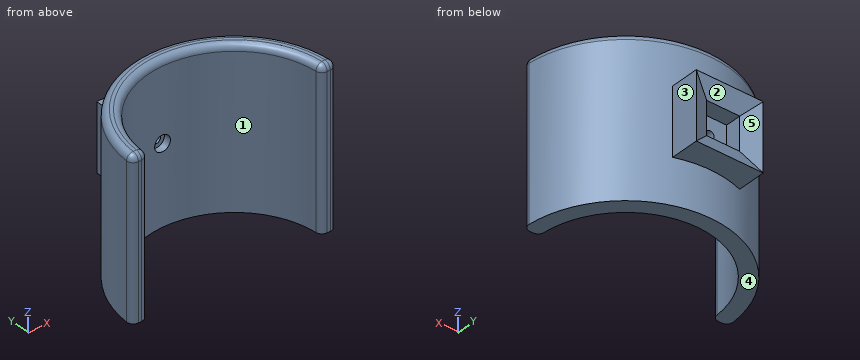
from build123d import *
from OCP.BRepFilletAPI import BRepFilletAPI_MakeChamfer

# Parameters (mm, degrees)
BOSS_EXTRUDE1_DEPTH = 50
BOSS_EXTRUDE2_DEPTH = 21.25
FILLET1_R           = 4
FILLET2_R           = 4
SKETCH3_W           = 21
SKETCH3_H           = 21
CUT_EXTRUDE1_DEPTH  = 15
CHAMFER1_SIZE       = 5
CHAMFER1_SIZE2      = 10.722534603
SKETCH4_R           = 2.5
CUT_EXTRUDE2_DEPTH  = 105.206319677
CUT_EXTRUDE3_START  = -5
SKETCH5_R           = 5
CUT_EXTRUDE3_DEPTH  = 100.206319725


with BuildPart() as part:
    # Sketch1 → Boss-Extrude1 (new, symmetric)
    with BuildSketch(Plane.XY):
        with BuildLine():
            Line((-65, 0), (-55, 0))
            ThreePointArc((-55, 0), (0, 55), (55, 0))
            Line((55, 0), (65, 0))
            ThreePointArc((65, 0), (0, 65), (-65, 0))
        make_face()
    extrude(amount=BOSS_EXTRUDE1_DEPTH, both=True)

    # Sketch2 → Boss-Extrude2 (add, symmetric)
    with BuildSketch(Plane.XY):
        with BuildLine():
            Line((-21.25, 61.428311877), (-21.25, 79.428311877))
            Line((-21.25, 79.428311877), (21.25, 79.428311877))
            Line((21.25, 79.428311877), (21.25, 61.428311877))
            ThreePointArc((21.25, 61.428311877), (0, 65), (-21.25, 61.428311877))
        make_face()
    extrude(amount=BOSS_EXTRUDE2_DEPTH, both=True)

    # Fillet1
    fillet1_edges = [part.edges().sort_by_distance(p)[0] for p in [
        (-55, 0, 0),
        (-65, 0, 0),
        (65, 0, 0),
        (55, 0, 0),
    ]]
    fillet(fillet1_edges, radius=FILLET1_R)

    # Fillet2
    fillet2_edges = [part.edges().sort_by_distance(p)[0] for p in [
        (0, 65, 50),
        (59.866480893, 0, 50),
        (0, 55, 50),
        (-59.866480893, 0, 50),
        (-63.788401254, 1.265880428, 50),
        (-56.133384976, 1.077266197, 50),
        (56.133384976, 1.077266197, 50),
        (63.788401254, 1.265880428, 50),
    ]]
    fillet(fillet2_edges, radius=FILLET2_R)

    # Sketch3 → Cut-Extrude1 (cut)
    with BuildSketch(Plane(origin=(0, 79.428311877, 0), x_dir=(1, 0, 0), z_dir=(0, 1, 0))):
        Rectangle(SKETCH3_W, SKETCH3_H)
    extrude(amount=-CUT_EXTRUDE1_DEPTH, mode=Mode.SUBTRACT)

    # Chamfer1: one chamfer whose edges measure the first distance from different faces: ONE call of the kernel's chamfer builder (chamfer() names one face for all edges)
    chamfer1_edges_1 = [part.edges().sort_by_distance(p)[0] for p in [
        (10.5, 79.428311877, 0),
    ]]
    chamfer1_side_1 = [part.faces().sort_by_distance(p)[0] for p in [
        (10.5, 71.928311877, 0),
    ]]
    chamfer1_edges_2 = [part.edges().sort_by_distance(p)[0] for p in [
        (0, 79.428311877, -10.5),
    ]]
    chamfer1_side_2 = [part.faces().sort_by_distance(p)[0] for p in [
        (0, 71.928311877, -10.5),
    ]]
    chamfer1_edges_3 = [part.edges().sort_by_distance(p)[0] for p in [
        (-10.5, 79.428311877, 0),
    ]]
    chamfer1_side_3 = [part.faces().sort_by_distance(p)[0] for p in [
        (-10.5, 71.928311877, 0),
    ]]
    chamfer1_edges_4 = [part.edges().sort_by_distance(p)[0] for p in [
        (0, 79.428311877, 10.5),
    ]]
    chamfer1_side_4 = [part.faces().sort_by_distance(p)[0] for p in [
        (0, 71.928311877, 10.5),
    ]]
    chamfer1 = BRepFilletAPI_MakeChamfer(part.part.solid().wrapped)
    for e in chamfer1_edges_1:
        chamfer1.Add(CHAMFER1_SIZE, CHAMFER1_SIZE2, e.wrapped, chamfer1_side_1[0].wrapped)  # the first distance lies on this face
    for e in chamfer1_edges_2:
        chamfer1.Add(CHAMFER1_SIZE, CHAMFER1_SIZE2, e.wrapped, chamfer1_side_2[0].wrapped)  # the first distance lies on this face
    for e in chamfer1_edges_3:
        chamfer1.Add(CHAMFER1_SIZE, CHAMFER1_SIZE2, e.wrapped, chamfer1_side_3[0].wrapped)  # the first distance lies on this face
    for e in chamfer1_edges_4:
        chamfer1.Add(CHAMFER1_SIZE, CHAMFER1_SIZE2, e.wrapped, chamfer1_side_4[0].wrapped)  # the first distance lies on this face
    add(Compound.cast(chamfer1.Shape()), mode=Mode.REPLACE)

    # Sketch4 → Cut-Extrude2 (cut, through all)
    with BuildSketch(Plane(origin=(0, 64.428311877, 0), x_dir=(1, 0, 0), z_dir=(0, 1, 0))):
        with Locations(Location((0, 0, 0), (0, 0, 270))):
            Circle(SKETCH4_R)
    extrude(amount=-CUT_EXTRUDE2_DEPTH, mode=Mode.SUBTRACT)

    # Sketch5 → Cut-Extrude3 (cut, through all)
    with BuildSketch(Plane(origin=(0, 64.428311877, 0), x_dir=(1, 0, 0), z_dir=(0, 1, 0)).offset(CUT_EXTRUDE3_START)):
        with Locations(Location((0, 0, 0), (0, 0, 270))):
            Circle(SKETCH5_R)
    extrude(amount=-CUT_EXTRUDE3_DEPTH, mode=Mode.SUBTRACT)


solid = part.part
Could you check a few things on this model? Use its own coordinates, in mm. Face numbers are marked on the shaded views. A direction names the side the tool comes from. Give positions to 0.01 mm unless a question says otherwise; leave off trailing zeros. Order: outer loops, then holes, each group sorted by start corner. A loop starts at its lowest first (then second) coordinate and runs counter-clockwise, first axis right, second up. Notation, with made-up numbers: (62, -15.5) -> (113, -15.5) arc R25 cw to (113, 13.5) -> close; hole circle Ø1 at (-5, 36). An arc over 180 degrees is marked (long way). Answer in a Markdown table with one row per item. Add a question column.
Item 1: For the marked faces 1 and 2, which set-ups out of +Z, -Z, +X, -X, +Y, -Y let a thin tool reach every point of the face, with its end or its side?
Item 2: I'm going to push flat-ended pins straight in: P1, Ø3, axis at x = -1.5, y = 69.5, coming from the +Z side; P2, Ø23, axis at x = -0.5, z = -5, coming from the +Y side; P3, Ø3, axis at x = 1.5, z = -0.5, coming from the -Y side. Where does each tip first touch, or does it pass through?
Item 3: We'd pull the mould along Z, two halves only. Please class the marked faces 3, 4 and 5: pulls with the +Z half, pulls with the -Z half, needs draft (parallel to the pull), parting line crosses it, or undercut.
Item 4: Please list where these lines run through material, in increasing order: probe 1 along X at (y, z) = (63.35, 0); probe 2 along X at (y, z) = (51, -26); probe 3 along Z at (x, y) = (0, 56.4).
Item 5: Imagine slicing it at C-C (y = 68). List the corners of the cut face in (x, z) for me.
Result:
| question | item | result |
|---|---|---|
| 1 | face 1 | +Z, -Z, -Y |
| 1 | face 2 | +Y |
| 2 | P1 | z = 21.25 |
| 2 | P2 | y = 77.23 |
| 2 | P3 | y = 59.43 |
| 3 | face 3 | needs draft |
| 3 | face 4 | pulls with the -Z half |
| 3 | face 5 | undercut |
| 4 | probe 1 | -21.25 to -2.5, 2.5 to 21.25 |
| 4 | probe 2 | -40.3 to -20.59, 20.59 to 40.3 |
| 4 | probe 3 | -50 to -5, 5 to 49.04 |
| 5 | outline | (-21.25, -21.25) -> (21.25, -21.25) -> (21.25, 21.25) -> (-21.25, 21.25) -> close; hole (-10.5, -10.5) -> (10.5, -10.5) -> (10.5, 10.5) -> (-10.5, 10.5) -> close |
